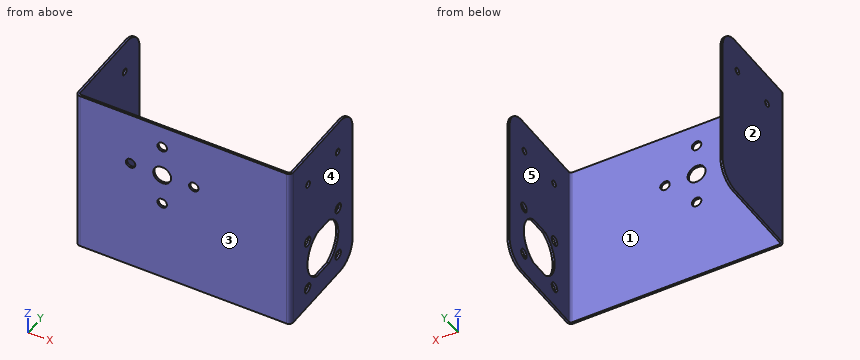
```python
from build123d import *

# Parameters (mm, degrees)
SKETCH1_W                    = 100
SKETCH1_H                    = 80
BASE_FLANGE1_DEPTH           = 1
EDGE_FLANGE1_STRIP_W         = 6
EDGE_FLANGE1_STRIP_H         = 1
EDGE_FLANGE1_STRIP_CUT_DEPTH = 80
EDGE_FLANGE1_DEPTH           = 80
EDGE_FLANGE2_STRIP_W         = 6
EDGE_FLANGE2_STRIP_H         = 1
EDGE_FLANGE2_STRIP_CUT_DEPTH = 80
EDGE_FLANGE2_DEPTH           = 80
FILLET1_R                    = 10
SKETCH12_R                   = 2.25
CUT_EXTRUDE1_DEPTH           = 10
SKETCH14_R                   = 4.25
SKETCH14_R_2                 = 2.25
CUT_EXTRUDE3_DEPTH           = 10
SKETCH15_R                   = 1.5
CUT_EXTRUDE4_DEPTH           = 167.440085507


# Sheet-metal steps are written as plain solids
with BuildPart() as part:
    # Sketch1 → Base-Flange1 (new body)
    with BuildSketch(Plane(origin=(0, 0, 0), x_dir=(1, 0, 0), z_dir=(0, 1, 0))):
        with Locations((50, 40)):
            Rectangle(SKETCH1_W, SKETCH1_H)
    extrude(amount=-BASE_FLANGE1_DEPTH)

    # Edge-Flange1 strip (across the edge) → Edge-Flange1 strip cut (cut)
    with BuildSketch(Plane(origin=(100, 0, 0), x_dir=(-1, 0, 0), z_dir=(0, 0, -1))):
        with Locations((-2, -0.5)):
            Rectangle(EDGE_FLANGE1_STRIP_W, EDGE_FLANGE1_STRIP_H)
    extrude(amount=EDGE_FLANGE1_STRIP_CUT_DEPTH, mode=Mode.SUBTRACT)

    # Edge-Flange1 section (across the edge) → Edge-Flange1 (add)
    with BuildSketch(Plane(origin=(100, 0, 0), x_dir=(-1, 0, 0), z_dir=(0, 0, -1))):
        with BuildLine():
            Line((-1, 1), (-1, 49))
            Line((-1, 49), (0, 49))
            Line((0, 49), (0, 1))
            ThreePointArc((0, 1), (0.292893219, 0.292893219), (1, 0))
            Line((1, 0), (1, -1))
            ThreePointArc((1, -1), (-0.414213562, -0.414213562), (-1, 1))
        make_face()
    extrude(amount=EDGE_FLANGE1_DEPTH)

    # Edge-Flange2 strip (across the edge) → Edge-Flange2 strip cut (cut)
    with BuildSketch(Plane.XY.offset(-80)):
        with Locations((-2, -0.5)):
            Rectangle(EDGE_FLANGE2_STRIP_W, EDGE_FLANGE2_STRIP_H)
    extrude(amount=EDGE_FLANGE2_STRIP_CUT_DEPTH, mode=Mode.SUBTRACT)

    # Edge-Flange2 section (across the edge) → Edge-Flange2 (add)
    with BuildSketch(Plane.XY.offset(-80)):
        with BuildLine():
            Line((-1, 1), (-1, 49))
            Line((-1, 49), (0, 49))
            Line((0, 49), (0, 1))
            ThreePointArc((0, 1), (0.292893219, 0.292893219), (1, 0))
            Line((1, 0), (1, -1))
            ThreePointArc((1, -1), (-0.414213562, -0.414213562), (-1, 1))
        make_face()
    extrude(amount=EDGE_FLANGE2_DEPTH)

    # Fillet1
    fillet1_edges = [part.edges().sort_by_distance(p)[0] for p in [
        (100.5, 49, 0),
        (100.5, 49, -80),
        (-0.5, 49, -80),
        (-0.5, 49, 0),
    ]]
    fillet(fillet1_edges, radius=FILLET1_R)

    # Sketch12 → Cut-Extrude1 (cut)
    with BuildSketch(Plane(origin=(101, 81.373526732, -102.532454166), x_dir=(0, 0, 1), z_dir=(1, 0, 0))):
        with BuildLine():
            ThreePointArc((56.332454166, 61.272506218), (44.832454166, 68.873526732), (33.332454166, 61.272506218))
            Line((33.332454166, 61.272506218), (33.332454166, 51.474547246))
            ThreePointArc((33.332454166, 51.474547246), (44.832454166, 43.873526732), (56.332454166, 51.474547246))
            Line((56.332454166, 51.474547246), (56.332454166, 61.272506218))
        make_face()
        with Locations(Location((32.458085495, 68.747895403, 0), (0, 0, 270))):
            Circle(SKETCH12_R)
        with Locations(Location((57.206822836, 68.747895403, 0), (0, 0, 270))):
            Circle(SKETCH12_R)
        with Locations(Location((57.206822836, 43.999158061, 0), (0, 0, 270))):
            Circle(SKETCH12_R)
        with Locations(Location((32.458085495, 43.999158061, 0), (0, 0, 270))):
            Circle(SKETCH12_R)
    extrude(amount=-CUT_EXTRUDE1_DEPTH, mode=Mode.SUBTRACT)

    # Sketch14 → Cut-Extrude3 (cut)
    with BuildSketch(Plane(origin=(82.686654231, -1, -102.532454166), x_dir=(-1, 0, 0), z_dir=(0, -1, 0))):
        with Locations(Location((42.686654231, -76.832454166, 0), (0, 0, 90))):
            Circle(SKETCH14_R)
        with Locations(Location((57.686654231, -76.832454166, 0), (0, 0, 90))):
            Circle(SKETCH14_R_2)
        with Locations(Location((42.686654231, -61.832454166, 0), (0, 0, 90))):
            Circle(SKETCH14_R_2)
        with Locations(Location((27.686654231, -76.832454166, 0), (0, 0, 90))):
            Circle(SKETCH14_R_2)
        with Locations(Location((42.686654231, -91.832454166, 0), (0, 0, 90))):
            Circle(SKETCH14_R_2)
    extrude(amount=-CUT_EXTRUDE3_DEPTH, mode=Mode.SUBTRACT)

    # Sketch15 → Cut-Extrude4 (cut, through all)
    with BuildSketch(Plane(origin=(101, 81.373526732, -102.532454166), x_dir=(0, 0, 1), z_dir=(1, 0, 0))):
        with Locations(Location((87.532454166, 44.373526732, 0), (0, 0, 270))):
            Circle(SKETCH15_R)
        with Locations(Location((87.532454166, 68.373526732, 0), (0, 0, 270))):
            Circle(SKETCH15_R)
    extrude(amount=-CUT_EXTRUDE4_DEPTH, mode=Mode.SUBTRACT)


solid = part.part
```
Verification items for the finished model (mm, model axes). Face numbers are marked on the shaded views. A direction names the side the tool comes from. Round coordinates to 2 decimals unless told otherwise and drop trailing zeros. Write each loop counter-clockwise with the first axis right and the second up, starting at its lowest first coordinate (ties: lowest second). Pieces come first, ordered by that corner, then holes. Notation, with made-up numbers: (42, -24) - (58, -24) arc R12 cw to (58, -18) - close; hole circle Ø7 at (-34.75, -14.5). An arc over 180 degrees is marked (long way). Answer as a JSON object with one key per item and string values. Group by question number.
Q1. Tool access check on the marked faces 4 and 5. Record the directions out of +Z, -Z, +X, -X, +Y, -Y that give a thin tool (end or side, any length) a straight path to the whole face; none if there is none.
Q2. Mould release check, pull along X, two halves, no side actions. Record for the marked faces 1, 2 and 3: released by +X, released by -X, zero draft, split by the parting line, or undercut.
Q3. Go/stop test with flat-tipped pins: pin 1 Ø6 at (x, z) = (12, -43.5) entering from +Y; pin 2 Ø1.8 at (y, z) = (37, -15) entering from +X; pin 3 Ø4 at (y, z) = (12.63, -70.07) entering from +X. Record where each tip stops, or that it passes through.
Q4. Section check D-D, the plane z = -25.7. Enter the section's corners in (x, y).
Q5. Thickness scan on line 1 (X direction, y = 7.5, z = -19.5); line 2 (Y direction, x = 63, z = -52.5); line 3 (X direction, y = -0.65, z = -40.7). Record the ranges inside material, lowest first.
Q6. Section check B-B, the plane z = -15. Enter the section's corners in (x, y).
Q7. Section check A-A, the plane x = 25. Enter the section's corners in (y, z).
Q8. Section check C-C, the plane y = 23. Enter the section's corners in (x, z), plus the area to 3 significant figures.
Found:
{
 "1": {"face 4": "+Z, -Z, +X, +Y, -Y", "face 5": "+Z, -Z, +Y"},
 "2": {"face 1": "undercut", "face 2": "released by -X", "face 3": "zero draft"},
 "3": {"pin 1": "stops at y = 0", "pin 2": "passes through", "pin 3": "stops at x = 0"},
 "4": {"outline": "(-1, 1) arc R2 ccw to (1, -1) - (22.75, -1) - (22.75, 0) - (1, 0) arc R1 cw to (0, 1) - (0, 49) - (-1, 49) - close; (27.25, -1) - (35.75, -1) - (35.75, 0) - (27.25, 0) - close; (44.25, -1) - (52.75, -1) - (52.75, 0) - (44.25, 0) - close; (57.25, -1) - (99, -1) arc R2 ccw to (101, 1) - (101, 49) - (100, 49) - (100, 1) arc R1 cw to (99, 0) - (57.25, 0) - close"},
 "5": {"line 1": "x = -1 to 0, 100 to 101", "line 2": "y = -1 to 0", "line 3": "x = -0.13 to 37.75, 42.25 to 100.13"},
 "6": {"outline": "(-1, 1) arc R2 ccw to (1, -1) - (99, -1) arc R2 ccw to (101, 1) - (101, 11.5) - (100, 11.5) - (100, 1) arc R1 cw to (99, 0) - (1, 0) arc R1 cw to (0, 1) - (0, 11.5) - (-1, 11.5) - close; (-1, 14.5) - (0, 14.5) - (0, 35.5) - (-1, 35.5) - close; (-1, 38.5) - (0, 38.5) - (0, 49) - (-1, 49) - close; (100, 14.5) - (101, 14.5) - (101, 35.5) - (100, 35.5) - close; (100, 38.5) - (101, 38.5) - (101, 49) - (100, 49) - close"},
 "7": {"outline": "(-1, -80) - (0, -80) - (0, -27.95) - (-1, -27.95) - close; (-1, -23.45) - (0, -23.45) - (0, 0) - (-1, 0) - close"},
 "8": {"outline": "(-1, -80) - (0, -80) - (0, 0) - (-1, 0) - close; (100, -80) - (101, -80) - (101, -69.2) - (100, -69.2) - close; (100, -46.2) - (101, -46.2) - (101, 0) - (100, 0) - close", "area": "137 mm^2"}
}
